Design review of the part built by this model. Coordinates are the model's own, in mm. Give positions to 0.01 mm unless a question says otherwise; leave off trailing zeros. Write each loop counter-clockwise with the first axis right and the second up, starting at its lowest first coordinate (ties: lowest second). Pieces come first, ordered by that corner, then holes. Notation, with made-up numbers: (52, 77.5) -> (101, 77.5) arc R15 ccw to (101, 101.5) -> close; hole circle Ø5 at (20.5, -17.75). An arc over 180 degrees is marked (long way). Answer as a JSON object with one key per item and string values.
```python
from build123d import *

# Parameters (mm, degrees)
BOSS_EXTRUDE1_DEPTH     = 10
CUT_EXTRUDE1_DEPTH      = 149.996644258
CUT_EXTRUDE1_DEPTH_BACK = 149.996644258
SKETCH2_R               = 17.5
SKETCH2_R_2             = 1.6
CUT_EXTRUDE2_DEPTH      = 149.996644258
CUT_EXTRUDE2_DEPTH_BACK = 149.996644258
SKETCH3_R               = 20
SKETCH3_R_2             = 2.6
CUT_EXTRUDE3_DEPTH      = 149.996644258
CUT_EXTRUDE3_DEPTH_BACK = 149.996644258
SKETCH4_R               = 1.6
FILLET1_R               = 10


with BuildPart() as part:
    # Sketch1 → Boss-Extrude1 (new body)
    with BuildSketch(Plane(origin=(0, 0, 0), x_dir=(1, 0, 0), z_dir=(0, 1, 0))):
        Polygon((-50, 60), (50, 60), (50, -80), (30, -80), (30, -140), (-30, -140), (-30, -80), (-50, -80), align=None)
    extrude(amount=BOSS_EXTRUDE1_DEPTH)

    # Sketch2 → Cut-Extrude1 (cut, two sides: drawn at the far end of the back side and taken through both)
    with BuildSketch(Plane(origin=(0, 10, 0), x_dir=(1, 0, 0), z_dir=(0, 1, 0)).offset(-CUT_EXTRUDE1_DEPTH_BACK)):
        with Locations(Location((0, 0, 0), (0, 0, 270))):
            Circle(SKETCH2_R)
        with Locations(Location((-40, -50, 0), (0, 0, 270))):
            Circle(SKETCH2_R_2)
        with Locations(Location((40, -50, 0), (0, 0, 270))):
            Circle(SKETCH2_R_2)
        with Locations(Location((40, 50, 0), (0, 0, 270))):
            Circle(SKETCH2_R_2)
        with Locations(Location((-40, 50, 0), (0, 0, 270))):
            Circle(SKETCH2_R_2)
        with Locations((-40, -130)):
            Circle(SKETCH2_R_2)
        with Locations((40, -130)):
            Circle(SKETCH2_R_2)
        with Locations((-40, -100)):
            Circle(SKETCH2_R_2)
        with Locations((40, -100)):
            Circle(SKETCH2_R_2)
    extrude(amount=CUT_EXTRUDE1_DEPTH + CUT_EXTRUDE1_DEPTH_BACK, mode=Mode.SUBTRACT)

    # Sketch3 → Cut-Extrude2 (cut, two sides: drawn at the far end of the back side and taken through both)
    with BuildSketch(Plane(origin=(0, 10, 0), x_dir=(1, 0, 0), z_dir=(0, 1, 0)).offset(-CUT_EXTRUDE2_DEPTH_BACK)):
        with Locations(Location((0, -110, 0), (0, 0, 270))):
            Circle(SKETCH3_R)
        with Locations(Location((-23.57, -86.43, 0), (0, 0, 270))):
            Circle(SKETCH3_R_2)
        with Locations(Location((23.57, -86.43, 0), (0, 0, 270))):
            Circle(SKETCH3_R_2)
        with Locations(Location((23.57, -133.57, 0), (0, 0, 270))):
            Circle(SKETCH3_R_2)
        with Locations(Location((-23.57, -133.57, 0), (0, 0, 270))):
            Circle(SKETCH3_R_2)
        with BuildLine():
            Line((-40, -66.8), (-10, -66.8))
            ThreePointArc((-10, -66.8), (-6.8, -70), (-10, -73.2))
            Line((-10, -73.2), (-40, -73.2))
            ThreePointArc((-40, -73.2), (-43.2, -70), (-40, -66.8))
        make_face()
        with BuildLine():
            Line((40, -66.8), (10, -66.8))
            ThreePointArc((10, -66.8), (6.8, -70), (10, -73.2))
            Line((10, -73.2), (40, -73.2))
            ThreePointArc((40, -73.2), (43.2, -70), (40, -66.8))
        make_face()
    extrude(amount=CUT_EXTRUDE2_DEPTH + CUT_EXTRUDE2_DEPTH_BACK, mode=Mode.SUBTRACT)

    # Sketch4 → Cut-Extrude3 (cut, two sides: drawn at the far end of the back side and taken through both)
    with BuildSketch(Plane(origin=(0, 10, 0), x_dir=(1, 0, 0), z_dir=(0, 1, 0)).offset(-CUT_EXTRUDE3_DEPTH_BACK)):
        with Locations(Location((-30, 10, 0), (0, 0, 270))):
            Circle(SKETCH4_R)
        with Locations(Location((-30, -10, 0), (0, 0, 270))):
            Circle(SKETCH4_R)
        with Locations(Location((30, 10, 0), (0, 0, 270))):
            Circle(SKETCH4_R)
        with Locations(Location((30, -10, 0), (0, 0, 270))):
            Circle(SKETCH4_R)
    extrude(amount=CUT_EXTRUDE3_DEPTH + CUT_EXTRUDE3_DEPTH_BACK, mode=Mode.SUBTRACT)

    # Fillet1
    fillet1_edges = [part.edges().sort_by_distance(p)[0] for p in [
        (50, 5, -60),
        (-50, 5, -60),
        (-30, 5, 80),
        (-30, 5, 140),
        (30, 5, 140),
        (30, 5, 80),
        (50, 5, 80),
        (-50, 5, 80),
    ]]
    fillet(fillet1_edges, radius=FILLET1_R - 0.0001)  # a hair under: the kernel refuses the full size


solid = part.part
```
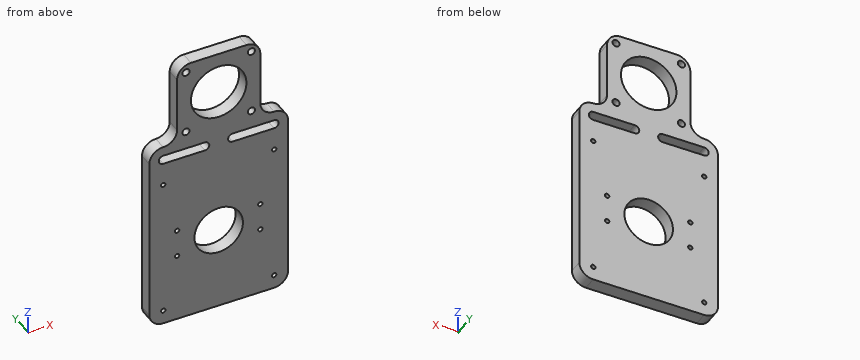
(1) We need section B-B, the plane x = 23.57. State the section outline as (y, z) points.
Here are the results:
{"outline": "(0, -60) -> (10, -60) -> (10, 66.8) -> (0, 66.8) -> close; (0, 73.2) -> (10, 73.2) -> (10, 83.83) -> (0, 83.83) -> close; (0, 89.03) -> (10, 89.03) -> (10, 130.97) -> (0, 130.97) -> close; (0, 136.17) -> (10, 136.17) -> (10, 139.34) -> (0, 139.34) -> close"}
(2) We need section A-A, the plane z = 110. State the section outline as (x, y) points, then the cut area to 3 significant figures.
Here are the results:
{"outline": "(-30, 0) -> (-20, 0) -> (-20, 10) -> (-30, 10) -> close; (20, 0) -> (30, 0) -> (30, 10) -> (20, 10) -> close", "area": "200 mm²"}
(3) We need section D-D, the plane y = 2.25. Give the number of separate pieces and of enclosed holes in the cut face, then the cut area to 3 significant figures.
Here are the results:
{"separate pieces": "1", "enclosed holes": "16", "area": "14,700 mm²"}
(4) Clearance check with a flat-ended pin moving along its axis: pin 1 (1 mm diameter, centred on y = 8, z = 116, fed in from +X). State where the tip first meets the part, or that it passes through.
Here are the results:
{"pin 1": "stops at x = 30"}
(5) We need section C-C, the plane z = 0.5. State the section outline as (x, y) points, then the cut area to 3 significant figures.
Here are the results:
{"outline": "(-50, 0) -> (-17.49, 0) -> (-17.49, 10) -> (-50, 10) -> close; (17.49, 0) -> (50, 0) -> (50, 10) -> (17.49, 10) -> close", "area": "650 mm²"}
(6) For line 1 along Z through (x, y) = (-40, 5.75); line 2 along Z through (x, y) = (0, 2.5); line 3 along X through (y, z) = (8, 50), list the stretches that pass through material, from the lowest coordinate up.
Here are the results:
{"line 1": "z = -60 to -51.6, -48.4 to 48.4, 51.6 to 66.8, 73.2 to 80", "line 2": "z = -60 to -17.5, 17.5 to 90, 130 to 140", "line 3": "x = -50 to -41.6, -38.4 to 38.4, 41.6 to 50"}
